Here's how the part is built. I have some questions about the finished solid (model axes, mm). A direction names the side the tool comes from. Coordinates: 2 decimals unless noted, no trailing zeros. Write each loop counter-clockwise with the first axis right and the second up, starting at its lowest first coordinate (ties: lowest second). Pieces come first, ordered by that corner, then holes. Notation, with made-up numbers: M 47,16.25 L 101,16.25 A7 cw 101,23.25 Z; hole C 21,-0.75 d7. An arc over 180 degrees is marked long. Use a Markdown table: item, result.
```python
from build123d import *

# Parameters (mm, degrees)
F3_D            = 5.5626
F3_COPIES_COUNT = 6
F4_R            = 2.54
F5_T            = 4.572


# Not quite as in the source:
# - a pattern or mirror of a feature is missing from the dataset's text; its kind, count and spacing are read off the source's solid
# - a shell that OpenCascade refuses in one call is made with other operations: the cavity is built on its own and cut out


with BuildPart() as f2:
    # F1 (on Front) → F2 (revolve)
    with BuildSketch(Plane.XZ):
        Polygon((25.4, 8.255), (0, 19.05), (0, -44.45), (25.4, -44.45), (25.4, 0), (40.64, 0), (40.64, 5.08), (25.4, 5.08), align=None)
    revolve(axis=Axis((0, 0, -12.7), (0, 0, 1)))

    # F3 (through all)
    with Locations(Plane(origin=(0, 0, 0), x_dir=(1, 0, 0), z_dir=(0, 0, -1))):
        with Locations((33.3375, 0)):
            f3 = Hole(F3_D / 2)

    # F3_copies: F3 ×6 about axis
    f3_copies_axis = Axis((0, 0, 0), (0, 0, 1))
    for i in range(1, F3_COPIES_COUNT):
        add(f3.rotate(f3_copies_axis, i * 360 / F3_COPIES_COUNT), mode=Mode.SUBTRACT)

    # F4
    f4_edges = [f2.edges().sort_by_distance(p)[0] for p in [
        (-25.4, 0, 8.255),
    ]]
    fillet(f4_edges, radius=F4_R)

    # F5: shell of thickness 4.572, made by hand


with BuildPart() as f5_core1:
    # F5_t2: copy of F2
    add(f2.part)

    # the walls: a layer under each face that stays
    f5_faces = [f5_core1.faces().sort_by_distance(p)[0] for p in [
        (-25.4, 0, 5.8273115729),
        (-24.9783818064, 0, 7.9760718686),
        (-27.0933333333, -27.0933333333, 5.08),
        (-11.9267486132, 0, 13.9811318394),
        (-40.64, 0, 2.54),
        (-15.2781, -26.4624454431, 2.54),
        (15.2781, -26.4624454431, 2.54),
        (30.5562, 0, 2.54),
        (-30.5562, 0, 2.54),
        (-15.2781, 26.4624454431, 2.54),
        (15.2781, 26.4624454431, 2.54),
        (27.0933333333, -27.0933333333, 0),
        (-25.4, 0, -22.225),
    ]]
    thicken(f5_faces, amount=-F5_T, mode=Mode.SUBTRACT)

    # F5_s3 → F5_t4 (revolve, cut)
    with BuildSketch(Plane.XZ):
        Polygon((25.44572, 5.12572), (20.828, 5.08), (20.828, 0.508), (25.4, 0.508), align=None)
    revolve(axis=Axis((0, 0, 5.08), (0, 0, 1)), mode=Mode.SUBTRACT)

    # F5_s5 → F5_t6 (revolve, cut)
    with BuildSketch(Plane.XZ):
        Polygon((25.44572, -0.04572), (25.4, 4.572), (20.828, 4.572), (20.828, 0), align=None)
    revolve(axis=Axis((0, 0, 0), (0, 0, 1)), mode=Mode.SUBTRACT)


with BuildPart() as f2_1:
    add(f2.part)

    # what is left inside the walls is the cavity
    f5_cavity = [f5_core1.part.solids().sort_by_distance(p)[0] for p in [
        (-20.78228, 0, -29.633333),
    ]]
    add(f5_cavity, mode=Mode.SUBTRACT)


solid = f2_1.part
```
1. Suppose I cut it at A-A on z = -28. Write out the boundary of the cut face in (x, y), and give its area (3 significant figures).
Answers follow:
| item | result |
|---|---|
| outline | C 0,0 d50.8; hole C 0,0 d41.66 |
| area | 664 mm2 |
2. I need wall thicknesses on probe 1 along X at (y, z) = (-0.5, -27.5); probe 2 along Z at (x, y) = (7, -36); probe 3 along Y at (x, z) = (33.5, 0.5). Which ranges of each line are inside material? Lowest first, please.
Answers follow:
| item | result |
|---|---|
| probe 1 | x = -25.4 to -20.82, 20.82 to 25.4 |
| probe 2 | z = 0 to 5.08 |
| probe 3 | y = -23.01 to -2.78, 2.78 to 23.01 |
3. We'd pull the mould along Y, two halves only. Please class faces 3 (the face through (-14.62, -30.75, 2.58)), 4 (the face through (-18.63, -17.49, 5.08)), 5 (the face through (13.65, 21.42, 5.84)): +Y half, -Y half, draft (parallel to the pull), parting line (faces both ways), or undercut.
Answers follow:
| item | result |
|---|---|
| face 3 | undercut |
| face 4 | draft |
| face 5 | parting line |
4. Which directions (+Z, -Z, +X, -X, +Y, -Y) give clear straight access to the entire face, cutting with the end or side of a thin tool? Please do faces 1 (the face through (13.89, 28.99, 2.58)), 2 (the face through (18.63, -17.49, 0)).
Answers follow:
| item | result |
|---|---|
| face 1 | +Z, -Z |
| face 2 | -Z |
5. Will these pins go through, and if not, where does the flat tip stop? pin 1 Ø6.5 at (x, y) = (-33.34, 0) entering from +Z; pin 2 Ø7 at (x, y) = (33.34, 0) entering from -Z; pin 3 Ø12 at (y, z) = (-20, 5.5) entering from -X.
Answers follow:
| item | result |
|---|---|
| pin 1 | stops at z = 5.08 |
| pin 2 | stops at z = 0 |
| pin 3 | stops at x = -38.15 |
